from build123d import *

# Parameters (mm, degrees)
BOSS_EXTRUDE1_DEPTH = 12.5
SKETCH5_W           = 10
SKETCH5_H           = 25
BOSS_EXTRUDE2_DEPTH = 25
SKETCH7_W           = 12
SKETCH7_H           = 30
BOSS_EXTRUDE4_DEPTH = 10.5
SKETCH8_R           = 6
CUT_EXTRUDE1_DEPTH  = 258.475083954
SKETCH11_W          = 16
SKETCH11_H          = 25
BOSS_EXTRUDE6_DEPTH = 10.5
SKETCH12_R          = 6.5
CUT_EXTRUDE3_DEPTH  = 356.26387941
SKETCH13_R          = 5
CUT_EXTRUDE4_DEPTH  = 261.08353454
FILLET2_R           = 30
FILLET3_R           = 5
FILLET4_R           = 5.5
CHAMFER1_SIZE       = 5
CHAMFER1_SIZE2      = 7


with BuildPart() as part:
    # Sketch2 → Boss-Extrude1 (new body)
    with BuildSketch(Plane(origin=(0, 0, 0), x_dir=(1, 0, 0), z_dir=(0, 1, 0))):
        Polygon((72.577488302, -150.138388534), (147.752897965, -177.5), (147.752897965, -207.5), (159.752897965, -207.5), (159.752897965, -177.5), (169.752897965, -177.5), (179.752897965, -177.5), (179.752897965, -207.5), (191.752897965, -207.5), (191.752897965, -177.5), (230.829328841, -150.138388534), (285.919436229, -50), (285.919436229, 0), (269.919436229, 0), (269.919436229, -25), (216.280811233, -122.5), (86.665258479, -122.5), (16, -25), (16, 0), (0, 0), (0, -50), align=None)
    extrude(amount=BOSS_EXTRUDE1_DEPTH)

    # Sketch5 → Boss-Extrude2 (add)
    with BuildSketch(Plane(origin=(0, 12.5, 0), x_dir=(1, 0, 0), z_dir=(0, 1, 0))):
        with Locations((157.252897965, -147.5)):
            Rectangle(SKETCH5_W, SKETCH5_H)
        with Locations((182.252897965, -147.5)):
            Rectangle(SKETCH5_W, SKETCH5_H)
    extrude(amount=BOSS_EXTRUDE2_DEPTH)

    # Sketch7 → Boss-Extrude4 (add)
    with BuildSketch(Plane(origin=(0, 12.5, 0), x_dir=(1, 0, 0), z_dir=(0, 1, 0))):
        with Locations((153.752897965, -192.5)):
            Rectangle(SKETCH7_W, SKETCH7_H)
        with Locations((185.752897965, -192.5)):
            Rectangle(SKETCH7_W, SKETCH7_H)
    extrude(amount=BOSS_EXTRUDE4_DEPTH)

    # Sketch8 → Cut-Extrude1 (cut, through all)
    with BuildSketch(Plane.ZY.offset(-147.752897965)):
        with Locations((192.5, 11.5)):
            Circle(SKETCH8_R)
    extrude(amount=-CUT_EXTRUDE1_DEPTH, mode=Mode.SUBTRACT)

    # Sketch11 → Boss-Extrude6 (add)
    with BuildSketch(Plane(origin=(0, 12.5, 0), x_dir=(1, 0, 0), z_dir=(0, 1, 0))):
        with Locations((8, -12.5)):
            Rectangle(SKETCH11_W, SKETCH11_H)
        with Locations((277.919436229, -12.5)):
            Rectangle(SKETCH11_W, SKETCH11_H)
    extrude(amount=BOSS_EXTRUDE6_DEPTH)

    # Sketch12 → Cut-Extrude3 (cut, through all)
    with BuildSketch(Plane.ZY):
        with Locations((12.5, 11.5)):
            Circle(SKETCH12_R)
    extrude(amount=-CUT_EXTRUDE3_DEPTH, mode=Mode.SUBTRACT)

    # Sketch13 → Cut-Extrude4 (cut, through all)
    with BuildSketch(Plane.ZY.offset(-152.252897965)):
        with Locations((147.5, 27.5)):
            Circle(SKETCH13_R)
    extrude(amount=-CUT_EXTRUDE4_DEPTH, mode=Mode.SUBTRACT)

    # Fillet2
    fillet2_edges = [part.edges().sort_by_distance(p)[0] for p in [
        (0, 6.25, 50),
        (86.665258479, 6.25, 122.5),
        (216.280811233, 6.25, 122.5),
        (285.919436229, 6.25, 50),
        (230.829328841, 6.25, 150.138388534),
        (72.577488302, 6.25, 150.138388534),
    ]]
    fillet(fillet2_edges, radius=FILLET2_R)

    # Fillet3
    fillet3_edges = [part.edges().sort_by_distance(p)[0] for p in [
        (185.752897965, 23, 207.5),
        (185.752897965, 23, 177.5),
        (8, 23, 25),
        (8, 23, 0),
        (277.919436229, 23, 25),
        (277.919436229, 23, 0),
        (157.252897965, 37.5, 160),
        (157.252897965, 37.5, 135),
        (182.252897965, 37.5, 160),
        (182.252897965, 37.5, 135),
        (153.752897965, 23, 207.5),
        (153.752897965, 23, 177.5),
    ]]
    fillet(fillet3_edges, radius=FILLET3_R)

    # Fillet4
    fillet4_edges = [part.edges().sort_by_distance(p)[0] for p in [
        (153.752897965, 12.5, 177.5),
        (185.752897965, 12.5, 177.5),
        (182.252897965, 12.5, 135),
        (157.252897965, 12.5, 135),
        (182.252897965, 12.5, 160),
        (157.252897965, 12.5, 160),
        (8, 12.5, 25),
        (277.919436229, 12.5, 25),
        (152.252897965, 12.5, 147.5),
        (187.252897965, 12.5, 147.5),
        (177.252897965, 12.5, 147.5),
        (162.252897965, 12.5, 147.5),
    ]]
    fillet(fillet4_edges, radius=FILLET4_R - 0.0001)  # a hair under: the kernel refuses the full size

    # Chamfer1
    chamfer1_edges = [part.edges().sort_by_distance(p)[0] for p in [
        (185.752897965, 0, 207.5),
        (153.752897965, 0, 207.5),
    ]]
    chamfer1_side = [part.faces().sort_by_distance(p)[0] for p in [
        (115.691812184, 0, 162.071200665),
    ]]
    chamfer(chamfer1_edges, length=CHAMFER1_SIZE, length2=CHAMFER1_SIZE2, reference=chamfer1_side[0])


solid = part.part
Part model, mm, in its own coordinate system. A direction names the side the tool comes from. Round coordinates to 2 decimals unless told otherwise and drop trailing zeros. Write each loop counter-clockwise with the first axis right and the second up, starting at its lowest first coordinate (ties: lowest second). Pieces come first, ordered by that corner, then holes. Notation, with made-up numbers: M 10.5,6.25 L 29.5,6.25 A9 cw 29.5,12.25 Z; hole C 50,39 d10. An arc over 180 degrees is marked long. Return JSON: item names as keys, results as strings. Group by question number.
(1) Two-plate mould, pull along Z, no slides. Class faces 1 (the face through (177.253, 23.3, 150.5)), 2 (the face through (182.4, 13.46, 132.605)), 3 (the face through (277.81, 13.45, 18.7)): +Z half, -Z half, draft (parallel to the pull), parting line (faces both ways), or undercut.
(2) Which spindle directions (+Z, -Z, +X, -X, +Y, -Y) get a long thin tool onto all of the face, cutting with end or side? Do faces 4 (the face through (162.253, 23.3, 150.5)), 5 (the face through (191.753, 6, 189)), 6 (the face through (187.61, 14.07, 175.85)), 7 (the face through (88.16, 6.34, 119.13)), 8 (the face through (154, 23, 192)). Say none if no direction does.
(3) Drill centre lines: probe 1 along Y at (x, z) = (9.25, 12.5); probe 2 along Z at (x, y) = (156, 11); probe 3 along Y at (x, z) = (188.5, 192.5). Where is each one in solid material? Low to high.
(4) Saw through at B-B on y = 27.5. Write the cut outline in (x, z), then the cut area to 3 significant figures.
(5) Saw through at D-D on x = 141. Write the cut outline in (y, z).
(6) Saw through at A-A on z = 12.5. Write the cut outline in (x, y), then the cut area to 3 significant figures.
(7) Pin check, flat tips, straight feed: pin 1 Ø13 at (x, z) = (154.5, 193.5) entering from +Y; pin 2 Ø4 at (x, y) = (163, 3.5) entering from -Z; pin 3 Ø15.5 at (y, z) = (11.5, 192.5) entering from +X. Stop position of each tip, or through.
(8) Saw through at C-C on z = 147.5. Write the cut outline in (x, y).
Returned:
{
 "1": {"face 1": "draft", "face 2": "-Z half", "face 3": "undercut"},
 "2": {"face 4": "+Z, -Z, +Y", "face 5": "+Z, +X, +Y, -Y", "face 6": "+X, -X, +Y", "face 7": "-Z, +Y, -Y", "face 8": "+Z, +X, -X, +Y"},
 "3": {"probe 1": "0 to 5, 18 to 23", "probe 2": "122.5 to 186.52, 198.48 to 207.5", "probe 3": "0 to 5.5, 17.5 to 23"},
 "4": {"outline": "M 152.25,135 L 162.25,135 L 162.25,142.5 L 152.25,142.5 Z; M 152.25,152.5 L 162.25,152.5 L 162.25,160 L 152.25,160 Z; M 177.25,135 L 187.25,135 L 187.25,142.5 L 177.25,142.5 Z; M 177.25,152.5 L 187.25,152.5 L 187.25,160 L 177.25,160 Z", "area": "300 mm²"},
 "5": {"outline": "M 0,122.5 L 12.5,122.5 L 12.5,172 A5.5 cw 13.42,175.04 L 0,175.04 Z"},
 "6": {"outline": "M 0,0 L 16,0 L 16,5 L 0,5 Z; M 0,18 L 16,18 L 16,23 L 0,23 Z; M 269.92,0 L 285.92,0 L 285.92,5 L 269.92,5 Z; M 269.92,18 L 285.92,18 L 285.92,23 L 269.92,23 Z", "area": "320 mm²"},
 "7": {"pin 1": "y = 23", "pin 2": "z = 122.5", "pin 3": "x = 191.75"},
 "8": {"outline": "M 71.53,0 L 231.96,0 L 231.96,12.5 L 192.75,12.5 A5.5 cw 187.25,18 L 187.25,22.5 L 177.25,22.5 L 177.25,18 A5.5 cw 171.75,12.5 L 167.75,12.5 A5.5 cw 162.25,18 L 162.25,22.5 L 152.25,22.5 L 152.25,18 A5.5 cw 146.75,12.5 L 71.53,12.5 Z; M 152.25,32.5 L 162.25,32.5 L 162.25,37.5 L 152.25,37.5 Z; M 177.25,32.5 L 187.25,32.5 L 187.25,37.5 L 177.25,37.5 Z"}
}
